Model file for the job. Use its own axes, mm. A direction names the side the tool comes from. Give positions to 0.01 mm unless a question says otherwise; leave off trailing zeros. Write each loop counter-clockwise with the first axis right and the second up, starting at its lowest first coordinate (ties: lowest second). Pieces come first, ordered by that corner, then holes. Notation, with made-up numbers: (65.25, 6.5) - (105.25, 6.5) arc R18 ccw to (105.25, 35.5) - close; hole circle Ø8 at (29, 62). An arc over 180 degrees is marked (long way). One line per item, written item: value. Start each with the question number.
(1) Probe L1, parallel to X at y = -8.5, z = 2.5; L2, parallel to Y at x = -3.5, z = 3.5; L3, parallel to Y at x = -3.25, z = 10.5. List the from-to ranges inside material, lowest first.
(2) Drop flat-ended pins along their axis: P1, Ø3, axis at y = 7.5, z = 17, coming from the -X side; P2, Ø0.9, axis at y = 7.5, z = -3, coming from the +X side; P3, Ø8, axis at x = -1.5, z = -4.5, coming from the -Y side; P4, Ø0.9, axis at x = -5, y = -10.65, coming from the -Z side. Give the stop position or say it passes through.
(3) 3-axis set-ups, long thin cutter, end or side, ignore diameter. For faces 1 (the face through (0, 7, 3)), 2 (the face through (-5, 7, -2)), 3 (the face through (5, 7, -3)): which of +Z, -Z, +X, -X, +Y, -Y reach the whole face in a straight line?
(4) Cut at C-C, the plane x = 7.75. List the corners of the cut face in (y, z).
(5) Mould opens along Z. For faces 4 (the face through (0, 5.65, 8)), 5 (the face through (-5, 7, 19)), 6 (the face through (-0.175, 20.035, 7.605)) say: pulls with the +Z half, pulls with the -Z half, needs draft (parallel to the pull), parting line crosses it, or undercut.
(6) Cut at B-B, the plane y = -13.5. List the corners of the cut face in (x, z), and give its area (3 significant figures).
(7) Cut at A-A, the plane x = -1. State how many separate pieces and enclosed holes the cut face has, and give its area (3 significant figures).
(8) Cut at D-D, the plane z = 12. List the corners of the cut face in (x, y), and give its area (3 significant figures).
from build123d import *

# Parameters (mm, degrees)
SKETCH1_W                = 25
SKETCH1_H                = 45
BOSS_EXTRUDE1_DEPTH      = 15
BOSS_EXTRUDE2_START      = -10.05
BOSS_EXTRUDE2_DEPTH      = 20.1
CUT_EXTRUDE1_DEPTH       = 30.79093822
CUT_EXTRUDE1_DEPTH_BACK  = 30.79093822
CUT_EXTRUDE3_DEPTH       = 30.79093822
CUT_EXTRUDE3_DEPTH_BACK  = 30.79093822
CUT_EXTRUDE7_DEPTH       = 30.79093822
CUT_EXTRUDE9_OUTLINE_W   = 21.12
CUT_EXTRUDE9_OUTLINE_H   = 10
CUT_EXTRUDE9_OUTLINE_W_2 = 21.100995898
CUT_EXTRUDE9_OUTLINE_H_2 = 2.85
CUT_EXTRUDE9_DEPTH       = 15
SKETCH8_W                = 7
SKETCH8_H                = 2.5
BOSS_EXTRUDE3_DEPTH      = 10
CUT_EXTRUDE11_DEPTH      = 30.79093822
CUT_EXTRUDE11_DEPTH_BACK = 30.79093822
CUT_EXTRUDE12_DEPTH      = 30.79093822
CUT_EXTRUDE12_DEPTH_BACK = 30.79093822
SKETCH10_R               = 1.6
CUT_EXTRUDE14_DEPTH      = 30.79093822
CUT_EXTRUDE14_DEPTH_BACK = 30.79093822
SKETCH12_R               = 0.75
CUT_EXTRUDE15_DEPTH      = 30.79093822
CUT_EXTRUDE15_DEPTH_BACK = 30.79093822
SKETCH15_W               = 15.416816506
SKETCH15_H               = 10.763431908
BOSS_EXTRUDE5_START      = 3
SKETCH16_W               = 21.100995898
SKETCH16_H               = 2.85
BOSS_EXTRUDE5_DEPTH      = 13
CUT_EXTRUDE17_DEPTH      = 30.79093822
CUT_EXTRUDE17_DEPTH_BACK = 30.79093822
SKETCH17_R               = 1.55
BOSS_EXTRUDE6_START      = 13
SKETCH18_W               = 21.100995898
SKETCH18_H               = 2.85
BOSS_EXTRUDE6_DEPTH      = 15
CUT_EXTRUDE18_DEPTH      = 39.032880511
CUT_EXTRUDE18_DEPTH_BACK = 39.032880511
SKETCH19_R               = 1.55


# Read off the part's stored shape, not the designer's step: Cut-Extrude9
with BuildPart() as part:
    # Sketch1 → Boss-Extrude1 (new body)
    with BuildSketch(Plane.XY):
        Rectangle(SKETCH1_W, SKETCH1_H)
    extrude(amount=BOSS_EXTRUDE1_DEPTH)

    # Sketch2 → Boss-Extrude2 (add)
    with BuildSketch(Plane(origin=(0, 0, 0), x_dir=(0, 0, -1), z_dir=(1, 0, 0)).offset(BOSS_EXTRUDE2_START)):
        Polygon((-15, 22.5), (-15, 21.775067879), (0, 22.5), align=None)
    extrude(amount=BOSS_EXTRUDE2_DEPTH)

    # Sketch3 → Cut-Extrude1 (cut, two sides: drawn at the far end of the back side and taken through both)
    with BuildSketch(Plane(origin=(0, 0, 0), x_dir=(0, 0, -1), z_dir=(1, 0, 0)).offset(-CUT_EXTRUDE1_DEPTH_BACK)):
        Polygon((-15, 22.5), (0, 17.5), (5.857225601, 19.69853849), (5.857225601, 28.456051758), (-15, 27.780768739), align=None)
    extrude(amount=CUT_EXTRUDE1_DEPTH + CUT_EXTRUDE1_DEPTH_BACK, mode=Mode.SUBTRACT)

    # Sketch4 → Cut-Extrude3 (cut, two sides: drawn at the far end of the back side and taken through both)
    with BuildSketch(Plane.XY.offset(-CUT_EXTRUDE3_DEPTH_BACK)):
        with BuildLine():
            Line((-17.124140969, -24.670147455), (0, -24.921234566))
            Line((0, -24.921234566), (0, -22.455047029))
            ThreePointArc((0, -22.455047029), (-8.838834765, -18.793881794), (-12.5, -9.955047029))
            Line((-12.5, -9.955047029), (-17.124140969, -24.670147455))
        make_face()
        with BuildLine():
            Line((0, -22.455047029), (0, -24.921234566))
            Line((0, -24.921234566), (18.053725517, -25.185951949))
            Line((18.053725517, -25.185951949), (12.5, -9.955047029))
            ThreePointArc((12.5, -9.955047029), (8.838834765, -18.793881794), (0, -22.455047029))
        make_face()
    extrude(amount=CUT_EXTRUDE3_DEPTH + CUT_EXTRUDE3_DEPTH_BACK, mode=Mode.SUBTRACT)

    # Sketch5 → Cut-Extrude7 (cut, through all)
    with BuildSketch(Plane.XY):
        with BuildLine():
            Line((10.560989946, -12.455047029), (-10.560989946, -12.455047029))
            ThreePointArc((-10.560989946, -12.455047029), (0, -20.455047029), (10.560989946, -12.455047029))
        make_face()
    extrude(amount=CUT_EXTRUDE7_DEPTH, mode=Mode.SUBTRACT)

    # Cut-Extrude9 outline → Cut-Extrude9 (cut)
    with BuildSketch(Plane.XY):
        with Locations((-0.129474346, -3.955047029)):
            Rectangle(CUT_EXTRUDE9_OUTLINE_W, CUT_EXTRUDE9_OUTLINE_H)
        with Locations((-0.010491997, 7.075)):
            Rectangle(CUT_EXTRUDE9_OUTLINE_W_2, CUT_EXTRUDE9_OUTLINE_H_2)
    extrude(amount=CUT_EXTRUDE9_DEPTH, mode=Mode.SUBTRACT)

    # Sketch8 → Boss-Extrude3 (add)
    with BuildSketch(Plane.XY):
        with Locations((0, 4.4)):
            Rectangle(SKETCH8_W, SKETCH8_H)
    extrude(amount=-BOSS_EXTRUDE3_DEPTH)

    # Sketch9 → Cut-Extrude11 (cut, two sides: drawn at the far end of the back side and taken through both)
    with BuildSketch(Plane(origin=(0, 0, 0), x_dir=(1, 0, 0), z_dir=(0, 1, 0)).offset(-CUT_EXTRUDE11_DEPTH_BACK)):
        with BuildLine():
            Line((-5.143587348, 10.809031185), (-3.492186712, 6.389631225))
            ThreePointArc((-3.492186712, 6.389631225), (0, 9.881817937), (3.492186712, 6.389631225))
            ThreePointArc((3.492186712, 6.389631225), (3.488488867, 6.228965567), (3.477403165, 6.068640163))
            Line((3.477403165, 6.068640163), (6.889064643, 10.549066481))
            Line((6.889064643, 10.549066481), (-5.143587348, 10.809031185))
        make_face()
    extrude(amount=CUT_EXTRUDE11_DEPTH + CUT_EXTRUDE11_DEPTH_BACK, mode=Mode.SUBTRACT)

    # Sketch10 → Cut-Extrude12 (cut, two sides: drawn at the far end of the back side and taken through both)
    with BuildSketch(Plane(origin=(0, 0, 0), x_dir=(1, 0, 0), z_dir=(0, 1, 0)).offset(-CUT_EXTRUDE12_DEPTH_BACK)):
        with Locations((0, 6.891628676)):
            Circle(SKETCH10_R)
        with BuildLine():
            ThreePointArc((1.6, 6.891628676), (0, 5.291628676), (-1.6, 6.891628676))
            Line((-1.6, 6.891628676), (-1.6, 0))
            Line((-1.6, 0), (1.6, 0))
            Line((1.6, 0), (1.6, 6.891628676))
        make_face()
    extrude(amount=CUT_EXTRUDE12_DEPTH + CUT_EXTRUDE12_DEPTH_BACK, mode=Mode.SUBTRACT)

    # Sketch12 → Cut-Extrude14 (cut, two sides: drawn at the far end of the back side and taken through both)
    with BuildSketch(Plane.XY.offset(-CUT_EXTRUDE14_DEPTH_BACK)):
        with Locations((-5, -10.646832198)):
            Circle(SKETCH12_R)
        with Locations((5, -10.646832198)):
            Circle(SKETCH12_R)
    extrude(amount=CUT_EXTRUDE14_DEPTH + CUT_EXTRUDE14_DEPTH_BACK, mode=Mode.SUBTRACT)

    # Sketch15 → Cut-Extrude15 (cut, two sides: drawn at the far end of the back side and taken through both)
    with BuildSketch(Plane(origin=(0, 0, 0), x_dir=(1, 0, 0), z_dir=(0, 1, 0)).offset(-CUT_EXTRUDE15_DEPTH_BACK)):
        with Locations((0.052797317, 5.381715954)):
            Rectangle(SKETCH15_W, SKETCH15_H)
    extrude(amount=CUT_EXTRUDE15_DEPTH + CUT_EXTRUDE15_DEPTH_BACK, mode=Mode.SUBTRACT)

    # Sketch16 → Boss-Extrude5 (add)
    with BuildSketch(Plane.XY.offset(BOSS_EXTRUDE5_START)):
        with Locations((-0.010491997, 7.075)):
            Rectangle(SKETCH16_W, SKETCH16_H)
    extrude(amount=-BOSS_EXTRUDE5_DEPTH)

    # Sketch17 → Cut-Extrude17 (cut, two sides: drawn at the far end of the back side and taken through both)
    with BuildSketch(Plane(origin=(0, 0, 0), x_dir=(1, 0, 0), z_dir=(0, 1, 0)).offset(-CUT_EXTRUDE17_DEPTH_BACK)):
        with Locations(Location((0, 6.400921521, 0), (0, 0, 270))):
            Circle(SKETCH17_R)
        with BuildLine():
            Line((5, 5), (5, 0))
            Line((5, 0), (12.5, 0))
            Line((12.5, 0), (12.436231279, 14.247241291))
            Line((12.436231279, 14.247241291), (-13.710360946, 14.247241291))
            Line((-13.710360946, 14.247241291), (-13.710360946, 0))
            Line((-13.710360946, 0), (-5, 0))
            Line((-5, 0), (-5, 5))
            ThreePointArc((-5, 5), (-3.535533906, 8.535533906), (0, 10))
            ThreePointArc((0, 10), (3.535533906, 8.535533906), (5, 5))
        make_face()
    extrude(amount=CUT_EXTRUDE17_DEPTH + CUT_EXTRUDE17_DEPTH_BACK, mode=Mode.SUBTRACT)

    # Sketch18 → Boss-Extrude6 (add)
    with BuildSketch(Plane.XY.offset(BOSS_EXTRUDE6_START)):
        with Locations((-0.010491997, 7.075)):
            Rectangle(SKETCH18_W, SKETCH18_H)
    extrude(amount=BOSS_EXTRUDE6_DEPTH)

    # Sketch19 → Cut-Extrude18 (cut, two sides: drawn at the far end of the back side and taken through both)
    with BuildSketch(Plane(origin=(0, 0, 0), x_dir=(1, 0, 0), z_dir=(0, 1, 0)).offset(-CUT_EXTRUDE18_DEPTH_BACK)):
        with Locations(Location((0, -24.160628435, 0), (0, 0, 270))):
            Circle(SKETCH19_R)
        with BuildLine():
            Line((-5, -23), (-5, -15))
            Line((-5, -15), (-19.938016683, -15))
            Line((-19.938016683, -15), (-19.938016683, -28.423127273))
            Line((-19.938016683, -28.423127273), (20.151320265, -28.423127273))
            Line((20.151320265, -28.423127273), (20.151320265, -15))
            Line((20.151320265, -15), (5, -15))
            Line((5, -15), (5, -23))
            ThreePointArc((5, -23), (0, -28), (-5, -23))
        make_face()
    extrude(amount=CUT_EXTRUDE18_DEPTH + CUT_EXTRUDE18_DEPTH_BACK, mode=Mode.SUBTRACT)


solid = part.part
Answers follow:
1. L1: x = -12.5 to -10.69, 10.43 to 12.5
1. L2: y = -21.96 to -19.88, -12.46 to -8.96, 1.04 to 5.65, 8.5 to 18.67
1. L3: y = -22.03 to -19.96, -12.46 to -8.96, 1.04 to 5.65, 8.5 to 21
2. P1: stops at x = -5
2. P2: stops at x = 5
2. P3: stops at y = 5.65
2. P4: passes through
3. face 1: none
3. face 2: -Z, -X, +Y, -Y
3. face 3: -Z, +X, +Y, -Y
4. outline: (-19.76, 0) - (-17.25, 0) - (-17.25, 15) - (-19.76, 15) - close; (-12.46, 0) - (-8.96, 0) - (-8.96, 15) - (-12.46, 15) - close; (1.04, 0) - (17.5, 0) - (22.5, 15) - (1.04, 15) - close; hole (5.65, 3) - (8.5, 3) - (8.5, 13) - (5.65, 13) - close
5. face 4: undercut
5. face 5: needs draft
5. face 6: pulls with the -Z half
6. outline: (-11.99, 0) - (-10.21, 0) - (-10.21, 15) - (-11.99, 15) - close; (10.21, 0) - (11.99, 0) - (11.99, 15) - (10.21, 15) - close
6. area: 53.3 mm²
7. separate pieces: 5
7. enclosed holes: 1
7. area: 390 mm²
8. outline: (-12.5, -9.96) arc R12.5 ccw to (12.5, -9.96) - (12.5, 21.5) - (-12.5, 21.5) - close; hole (-10.69, -8.96) - (10.43, -8.96) - (10.43, 1.04) - (-10.69, 1.04) - close; hole (-10.56, -12.46) arc R10.97 ccw to (10.56, -12.46) - close; hole (-10.56, 5.65) - (10.54, 5.65) - (10.54, 8.5) - (-10.56, 8.5) - close; hole circle Ø1.5 at (-5, -10.65); hole circle Ø1.5 at (5, -10.65)
8. area: 632 mm²
